```python
from build123d import *

# Parameters (mm, degrees)
SKETCH1_R           = 34.464858416
SKETCH1_R_2         = 2.15
SKETCH1_R_3         = 7.62
BOSS_EXTRUDE1_DEPTH = 4.7625


with BuildPart() as part:
    # Sketch1 → Boss-Extrude1 (new body)
    with BuildSketch(Plane(origin=(0, 0, 0), x_dir=(1, 0, 0), z_dir=(0, 1, 0))):
        with Locations((0, -8.264651725)):
            Circle(SKETCH1_R)
        with Locations((15, -8.264651725)):
            Circle(SKETCH1_R_2, mode=Mode.SUBTRACT)
        with Locations((22, -8.264651725)):
            Circle(SKETCH1_R_2, mode=Mode.SUBTRACT)
        with Locations((0, -23.264651725)):
            Circle(SKETCH1_R_2, mode=Mode.SUBTRACT)
        with Locations((0, -30.264651725)):
            Circle(SKETCH1_R_2, mode=Mode.SUBTRACT)
        with Locations((-15, -8.264651725)):
            Circle(SKETCH1_R_2, mode=Mode.SUBTRACT)
        with Locations((-22, -8.264651725)):
            Circle(SKETCH1_R_2, mode=Mode.SUBTRACT)
        with Locations((0, 6.735348275)):
            Circle(SKETCH1_R_2, mode=Mode.SUBTRACT)
        with Locations((0, 13.735348275)):
            Circle(SKETCH1_R_2, mode=Mode.SUBTRACT)
        with Locations((0, -8.264651725)):
            Circle(SKETCH1_R_3, mode=Mode.SUBTRACT)
    extrude(amount=BOSS_EXTRUDE1_DEPTH)


solid = part.part
```
Part model, mm, in its own coordinate system. Round coordinates to 2 decimals unless told otherwise and drop trailing zeros. Loops run counter-clockwise (first coordinate to the right, second up) from the corner with the lowest first, then second, coordinate; pieces in that order, holes last. Notation, with made-up numbers: (-31.75, 33.25) -> (6.25, 33.25) arc R22 cw to (6.25, 65.25) -> close; hole circle Ø11 at (36, -19.5). An arc over 180 degrees is marked (long way). Use one line per item in the form item = value. Start each with the question number.
Item 1: Two-plate mould, pull along X, no slides. Class faces 1 (the cylindrical face through (19.852, 2.348, 8.17)), 2 (the flat face through (0, 0, 0)), 3 (the cylindrical face through (-25.4, 2.35, -15.03)): released by +X, released by -X, zero draft, split by the parting line, or undercut.
Item 2: Drop a flat-ended pin along its axis: pin 1 Ø1.5 at (x, z) = (19, 0.5) entering from -Y. Give the stop position or say it passes through.
Item 3: Band-saw the part on D-D (y = 2.05). Give the number of separate pieces and of enclosed holes in the cut face, plus the area to 3 significant figures.
Item 4: Band-saw the part on B-B (z = 31.5). List the corners of the cut face in (x, y).
Item 5: Drill centre lines: line 1 along Z through (x, y) = (0, 3.3); line 2 along X through (y, z) = (2.15, -5); line 3 along X through (y, z) = (1.75, 10.5). Where is each one in solid material? Low to high.
Item 6: Band-saw the part on C-C (x = 22). List the corners of the cut face in (y, z), plus the area to 3 significant figures.
Item 7: Band-saw the part on A-A (x = 0). List the corners of the cut face in (y, z), plus the area to 3 significant figures.
Data:
q1.face_1 = undercut
q1.face_2 = zero draft
q1.face_3 = split by the parting line
q2.pin_1 = 0
q3.separate_pieces = 1
q3.enclosed_holes = 9
q3.area = 3,430 mm^2
q4.outline = (-25.45, 0) -> (-1.76, 0) -> (-1.76, 4.76) -> (-25.45, 4.76) -> close; (1.76, 0) -> (25.45, 0) -> (25.45, 4.76) -> (1.76, 4.76) -> close
q5.line_1 = -26.2 to -15.89, -11.59 to -8.89, -4.59 to 0.64, 15.88 to 21.11, 25.41 to 28.11, 32.41 to 42.73
q5.line_2 = -31.81 to -1.27, 1.27 to 31.81
q5.line_3 = -34.39 to -7.28, 7.28 to 34.39
q6.outline = (0, -18.27) -> (4.76, -18.27) -> (4.76, 6.11) -> (0, 6.11) -> close; (0, 10.41) -> (4.76, 10.41) -> (4.76, 34.79) -> (0, 34.79) -> close
q6.area = 232 mm^2
q7.outline = (0, -26.2) -> (4.76, -26.2) -> (4.76, -15.89) -> (0, -15.89) -> close; (0, -11.59) -> (4.76, -11.59) -> (4.76, -8.89) -> (0, -8.89) -> close; (0, -4.59) -> (4.76, -4.59) -> (4.76, 0.64) -> (0, 0.64) -> close; (0, 15.88) -> (4.76, 15.88) -> (4.76, 21.11) -> (0, 21.11) -> close; (0, 25.41) -> (4.76, 25.41) -> (4.76, 28.11) -> (0, 28.11) -> close; (0, 32.41) -> (4.76, 32.41) -> (4.76, 42.73) -> (0, 42.73) -> close
q7.area = 174 mm^2
